Can you work these out from the model? Positions are in its coordinate system, mm. Give positions to 0.01 mm unless a question says otherwise; leave off trailing zeros. Order: outer loops, then holes, each group sorted by start corner. A loop starts at its lowest first (then second) coordinate and runs counter-clockwise, first axis right, second up. Notation, with made-up numbers: (-0.5, -32.5) - (3.5, -32.5) arc R17 ccw to (3.5, -22.5) - close; hole circle Ø11 at (23.5, 77.25). An arc over 180 degrees is marked (long way). One line per question, with ' | ' between items.
```python
from build123d import *

# Parameters (mm, degrees)
SZKIC1_W                    = 56.4
SZKIC1_H                    = 80
DODANIE_WYCI_GNI_CIE1_DEPTH = 5
OTWORY_USTALAJ_CE_4_0MM1_D  = 4


with BuildPart() as part:
    # Szkic1 → Dodanie-wyciągnięcie1 (new body)
    with BuildSketch(Plane(origin=(0, 0, 0), x_dir=(0, 0, -1), z_dir=(1, 0, 0))):
        with Locations((28.2, 40)):
            Rectangle(SZKIC1_W, SZKIC1_H)
    extrude(amount=DODANIE_WYCI_GNI_CIE1_DEPTH)

    # Otwory ustalające Ø4.0mm1 (through all)
    with Locations(Plane(origin=(2.5, 80, -51.77), x_dir=(0, 0, 1), z_dir=(0, 1, 0))):
        with Locations((0, 0), (47.14, 0)):
            Hole(OTWORY_USTALAJ_CE_4_0MM1_D / 2)


solid = part.part
```
(1) If I drill on line 1 (Z direction, x = 2.65, y = 69); line 2 (X direction, y = 33, z = -51.5); line 3 (Z direction, x = 3.8, y = 46.5), over which ranges is the centre line in solid material (lowest first)?
Answer below:
line 1: -56.4 to -53.76, -49.78 to -6.62, -2.64 to 0 | line 2: 0 to 0.52, 4.48 to 5 | line 3: -56.4 to -53.29, -50.25 to -6.15, -3.11 to 0
(2) If we mould it in two halves opening along X, with no side actions, what happens to faces 1 (the face through (2, 80, -28)), 2 (the face through (5, 41, -28)), 3 (the face through (1.283, 39.44, -3.043))? For each: released by +X, released by -X, zero draft, split by the parting line, or undercut.
Answer below:
face 1: zero draft | face 2: released by +X | face 3: undercut
(3) Imagine slicing it at B-B (y = 74). List the corners of the cut face in (x, z) for me.
Answer below:
outline: (0, -56.4) - (5, -56.4) - (5, 0) - (0, 0) - close; hole circle Ø4 at (2.5, -51.77); hole circle Ø4 at (2.5, -4.63)
(4) Imagine slicing it at A-A (z = -51.77). List the corners of the cut face in (x, y) for me.
Answer below:
outline: (0, 0) - (0.5, 0) - (0.5, 80) - (0, 80) - close; (4.5, 0) - (5, 0) - (5, 80) - (4.5, 80) - close
(5) Imagine slicing it at C-C (x = 1.3). List the corners of the cut face in (y, z) for me.
Answer below:
outline: (0, -56.4) - (80, -56.4) - (80, -53.37) - (0, -53.37) - close; (0, -50.17) - (80, -50.17) - (80, -6.23) - (0, -6.23) - close; (0, -3.03) - (80, -3.03) - (80, 0) - (0, 0) - close
